from build123d import *

# Parameters (mm, degrees)
SKETCH1_W           = 500
SKETCH1_H           = 40
BOSS_EXTRUDE1_DEPTH = 3
SKETCH3_W           = 50
SKETCH3_H           = 20
CUT_EXTRUDE2_DEPTH  = 4


with BuildPart() as part:
    # Sketch1 → Boss-Extrude1 (new body)
    with BuildSketch(Plane.XY):
        with Locations((250, 20)):
            Rectangle(SKETCH1_W, SKETCH1_H)
    extrude(amount=BOSS_EXTRUDE1_DEPTH)

    # Sketch3 → Cut-Extrude2 (cut, through all)
    with BuildSketch(Plane.XY.offset(3)):
        with Locations((75, 30)):
            Rectangle(SKETCH3_W, SKETCH3_H)
        with Locations((150, 30)):
            Rectangle(SKETCH3_W, SKETCH3_H)
        with Locations((250, 30)):
            Rectangle(SKETCH3_W, SKETCH3_H)
        with Locations((425, 30)):
            Rectangle(SKETCH3_W, SKETCH3_H)
        with Locations((350, 30)):
            Rectangle(SKETCH3_W, SKETCH3_H)
    extrude(amount=-CUT_EXTRUDE2_DEPTH, mode=Mode.SUBTRACT)


solid = part.part
Can you work these out from the model? Positions are in its coordinate system, mm. Give positions to 0.01 mm unless a question says otherwise; leave off trailing zeros. Loops run counter-clockwise (first coordinate to the right, second up) from the corner with the lowest first, then second, coordinate; pieces in that order, holes last. Notation, with made-up numbers: M 37,71.5 L 86,71.5 A31 ccw 86,97.5 Z; hole C 4,33.25 d4. An arc over 180 degrees is marked long. One line per item, written item: value.
1) Imagine slicing it at B-B on z = 1.7. Write out the boundary of the cut face in (x, y), and give its area (3 significant figures).
Geometry check:
outline: M 0,0 L 500,0 L 500,40 L 450,40 L 450,20 L 400,20 L 400,40 L 375,40 L 375,20 L 325,20 L 325,40 L 275,40 L 275,20 L 225,20 L 225,40 L 175,40 L 175,20 L 125,20 L 125,40 L 100,40 L 100,20 L 50,20 L 50,40 L 0,40 Z
area: 15,000 mm²
2) I'm going to push a flat-ended pin straight in: pin 1 (0.9 mm diameter, centred on x = 142.5, z = 1.5, fed in from +Y). Where does the tip first touch, or does it pass through?
Geometry check:
pin 1: stops at y = 20
3) Imagine slicing it at A-A on y = 26.5. Write out the boundary of the cut face in (x, z).
Geometry check:
outline: M 0,0 L 50,0 L 50,3 L 0,3 Z; M 100,0 L 125,0 L 125,3 L 100,3 Z; M 175,0 L 225,0 L 225,3 L 175,3 Z; M 275,0 L 325,0 L 325,3 L 275,3 Z; M 375,0 L 400,0 L 400,3 L 375,3 Z; M 450,0 L 500,0 L 500,3 L 450,3 Z
4) Imagine slicing it at C-C on x = 72.5. Write out the boundary of the cut face in (y, z).
Geometry check:
outline: M 0,0 L 20,0 L 20,3 L 0,3 Z
5) Please list where these lines run through material, in increasing order: line 1 (X direction, y = 29.5, z = 0.75); line 2 (Y direction, x = 235.5, z = 2.25).
Geometry check:
line 1: x = 0 to 50, 100 to 125, 175 to 225, 275 to 325, 375 to 400, 450 to 500
line 2: y = 0 to 20
